from build123d import *

# Parameters (mm, degrees)
ESQUISSE1_R                             = 15
BOSS_EXTRU_1_DEPTH                      = 2
ESQUISSE2_R                             = 15
ESQUISSE2_R_2                           = 13
BOSS_EXTRU_2_DEPTH                      = 1
ESQUISSE3_R                             = 15
ESQUISSE3_R_2                           = 12.5
BOSS_EXTRU_3_DEPTH                      = 6
ESQUISSE5_R                             = 8.5
ENL_V_MAT_EXTRU_1_DEPTH                 = 0.5
ESQUISSE6_R                             = 7
ENL_V_MAT_EXTRU_2_DEPTH                 = 1.5
DIAM_TRE_DU_PER_AGE_2_0_2_1_D           = 2
DIAM_TRE_DU_PER_AGE_2_0_2_1_CSINK_D     = 2.05
DIAM_TRE_DU_PER_AGE_2_0_2_1_CSINK_ANGLE = 90


with BuildPart() as part:
    # Esquisse1 → Boss.-Extru.1 (new body)
    with BuildSketch(Plane.XY):
        Circle(ESQUISSE1_R)
    extrude(amount=BOSS_EXTRU_1_DEPTH)

    # Esquisse2 → Boss.-Extru.2 (add)
    with BuildSketch(Plane.XY.offset(2)):
        Circle(ESQUISSE2_R)
        Circle(ESQUISSE2_R_2, mode=Mode.SUBTRACT)
    extrude(amount=BOSS_EXTRU_2_DEPTH)

    # Esquisse3 → Boss.-Extru.3 (add)
    with BuildSketch(Plane.XY.offset(3)):
        Circle(ESQUISSE3_R)
        Circle(ESQUISSE3_R_2, mode=Mode.SUBTRACT)
    extrude(amount=BOSS_EXTRU_3_DEPTH)

    # Esquisse5 → Enlèv. mat.-Extru.1 (cut)
    with BuildSketch(Plane(origin=(0, 0, 0), x_dir=(-1, 0, 0), z_dir=(0, 0, -1))):
        Circle(ESQUISSE5_R)
    extrude(amount=-ENL_V_MAT_EXTRU_1_DEPTH, mode=Mode.SUBTRACT)

    # Esquisse6 → Enlèv. mat.-Extru.2 (cut)
    with BuildSketch(Plane(origin=(0, 0, 0.5), x_dir=(-1, 0, 0), z_dir=(0, 0, -1))):
        Circle(ESQUISSE6_R)
    extrude(amount=-ENL_V_MAT_EXTRU_2_DEPTH, mode=Mode.SUBTRACT)

    # Diamètre du perçage Ø2.0 (2)1 (through all)
    with Locations(Plane(origin=(0, 0, 0), x_dir=(-1, 0, 0), z_dir=(0, 0, -1))):
        with Locations((0, -10.5), (0, 10.5)):
            CounterSinkHole(DIAM_TRE_DU_PER_AGE_2_0_2_1_D / 2, DIAM_TRE_DU_PER_AGE_2_0_2_1_CSINK_D / 2, counter_sink_angle=DIAM_TRE_DU_PER_AGE_2_0_2_1_CSINK_ANGLE)


solid = part.part
Verification items for the finished model (mm, model axes). A direction names the side the tool comes from. Coordinates: 2 decimals unless noted, no trailing zeros. Order: outer loops, then holes, each group sorted by start corner. A loop starts at its lowest first (then second) coordinate and runs counter-clockwise, first axis right, second up. Notation, with made-up numbers: M 12.25,88 L 37.25,88 A20 cw 37.25,117 Z; hole C 10.5,26 d7. An arc over 180 degrees is marked long. One line per item, written item: value. Start each with the question number.
Item 1: Scan lines: probe 1 along Y at (x, z) = (0, 0.25); probe 2 along Y at (x, z) = (0, 6.4); probe 3 along Z at (x, y) = (12.5, 3.25). Record each from-to range of solid material in increasing order.
Item 2: Access from +Z, -Z, +X, -X, +Y, -Y to the whole of each face (thin tool, end or side, straight path). Record for faces 5 (the flat face through (-6.8, 10.7, 3)), 6 (the flat face through (6.5, -6.5, 0)), 7 (the flat face through (-2, 7, 0.5)), 8 (the cylindrical face through (-0.13, -9.51, 1.03)), 9 (the cylindrical face through (11.923, 3.755, 5.958)).
Item 3: Sectioned sample at B-B (y = 0). Enter the section's corners in (x, z), then the cut area to 3 significant figures.
Item 4: Mould release check, pull along Y, two halves, no side actions. Record for faces 1 (the cylindrical face through (-4.57, 7.167, 0.246)), 2 (the flat face through (6, -6, 2)), 3 (the flat face through (-3.4, 12.3, 9)), 4 (the cylindrical face through (-14.985, 0.66, 4.437)): released by +Y, released by -Y, zero draft, split by the parting line, or undercut.
Item 5: Gauge pin test, flat ends, axial feed: pin 1 (15.5 mm diameter, centred on x = 0, y = 0, fed in from -Z); pin 2 (3 mm diameter, centred on x = -8.5, z = 7, fed in from -Y); pin 3 (4 mm diameter, centred on x = -2.5, z = 2.5, fed in from -Y); pin 4 (1.8 mm diameter, centred on x = 0, y = -10.5, fed in from +Z). Record the tip position at first contact, or that the pin passes through.
Item 6: Sectioned sample at A-A (x = 5.25). Enter the section's corners in (y, z).
Item 7: Sectioned sample at C-C (x = 0). Count the separate pieces of the cut face and the enclosed holes in it, then the cut area to 3 significant figures.
Item 8: Sectioned sample at D-D (z = 5). Enter the section's corners in (x, y).
Conclusion:
1. probe 1: y = -15 to -11.5, -9.5 to -8.5, 8.5 to 9.5, 11.5 to 15
1. probe 2: y = -15 to -12.5, 12.5 to 15
1. probe 3: z = 0 to 2, 3 to 9
2. face 5: none
2. face 6: -Z, +X, -X, +Y, -Y
2. face 7: -Z
2. face 8: +Z, -Z
2. face 9: +Z
3. outline: M -15,0 L -8.5,0 L -8.5,0.5 L -7,0.5 L -7,2 L -13,2 L -13,3 L -12.5,3 L -12.5,9 L -15,9 Z; M 7,0.5 L 8.5,0.5 L 8.5,0 L 15,0 L 15,9 L 12.5,9 L 12.5,3 L 13,3 L 13,2 L 7,2 Z
3. area: 64.5 mm^2
4. face 1: undercut
4. face 2: undercut
4. face 3: zero draft
4. face 4: split by the parting line
5. pin 1: stops at z = 0.5
5. pin 2: stops at y = -13.27
5. pin 3: stops at y = -14.99
5. pin 4: passes through
6. outline: M -14.05,0 L -6.68,0 L -6.68,0.5 L -4.63,0.5 L -4.63,2 L -11.89,2 L -11.89,3 L -11.34,3 L -11.34,9 L -14.05,9 Z; M 4.63,0.5 L 6.68,0.5 L 6.68,0 L 14.05,0 L 14.05,9 L 11.34,9 L 11.34,3 L 11.89,3 L 11.89,2 L 4.63,2 Z
7. separate pieces: 4
7. enclosed holes: 0
7. area: 56.5 mm^2
8. outline: C 0,0 d30; hole C 0,0 d25
